Here's the drawing with two shaded views (mm, measured from the low corner). I have some questions. A direction names the side the tool comes from. Give positions to 0.01 mm unless a question says otherwise; leave off trailing zeros. Loops run counter-clockwise (first coordinate to the right, second up) from the corner with the lowest first, then second, coordinate; pieces in that order, holes last.
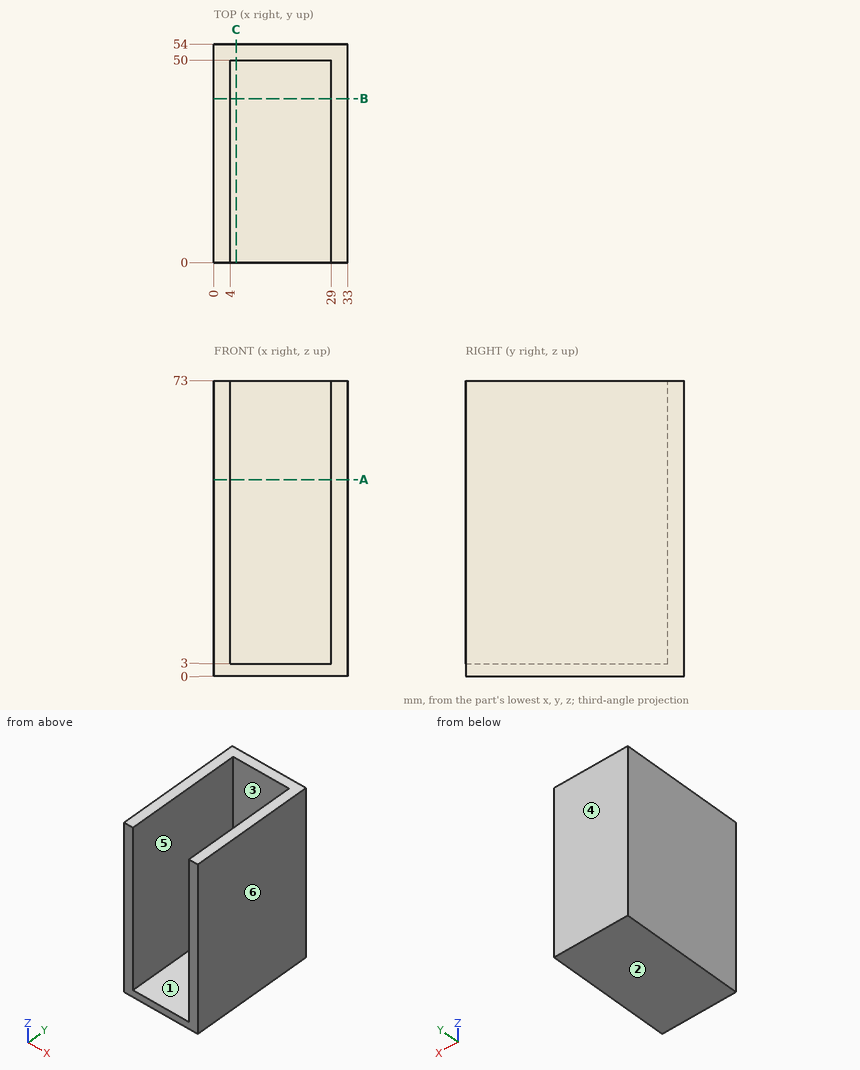
(1) Which directions (+Z, -Z, +X, -X, +Y, -Y) give clear straight access to the entire face, cutting with the end or side of a thin tool? Please do the marked faces 1 and 2.
Returned:
face 1: +Z, -Y
face 2: -Z, +X, -X, +Y, -Y
(2) Please list where these lines run through material, in increasing order: probe 1 along X at (y, z) = (14.5, 45.5); probe 2 along Y at (x, z) = (7.5, 39); probe 3 along Z at (x, y) = (20, 17.5).
Returned:
probe 1: x = 0 to 4, 29 to 33
probe 2: y = 50 to 54
probe 3: z = 0 to 3
(3) Thinking about a two-plate mould opening in X: for the marked faces 3, 4, 5 and 6, which applies, pulls with the +X half, pulls with the -X half, needs draft (parallel to the pull), parting line crosses it, or undercut?
Returned:
face 3: undercut
face 4: needs draft
face 5: undercut
face 6: pulls with the +X half
(4) Suppose I cut it at C-C on x = 5.5. List the corners of the cut face in (y, z) for me.
Returned:
outline: (0, 0) - (54, 0) - (54, 73) - (50, 73) - (50, 3) - (0, 3) - close
(5) Will these pins go through, and if not, where does the flat tip stop? P1, Ø1.5, axis at x = 15.5, z = 20.5, coming from the -Y side; P2, Ø1, axis at x = 15, y = 18, coming from the +Z side.
Returned:
P1: stops at y = 50
P2: stops at z = 3
(6) Suppose I cut it at A-A on z = 48.5. List the corners of the cut face in (x, y) for me.
Returned:
outline: (0, 0) - (4, 0) - (4, 50) - (29, 50) - (29, 0) - (33, 0) - (33, 54) - (0, 54) - close
(7) Suppose I cut it at B-B on y = 40.5. List the corners of the cut face in (x, z) for me.
Returned:
outline: (0, 0) - (33, 0) - (33, 73) - (29, 73) - (29, 3) - (4, 3) - (4, 73) - (0, 73) - close
